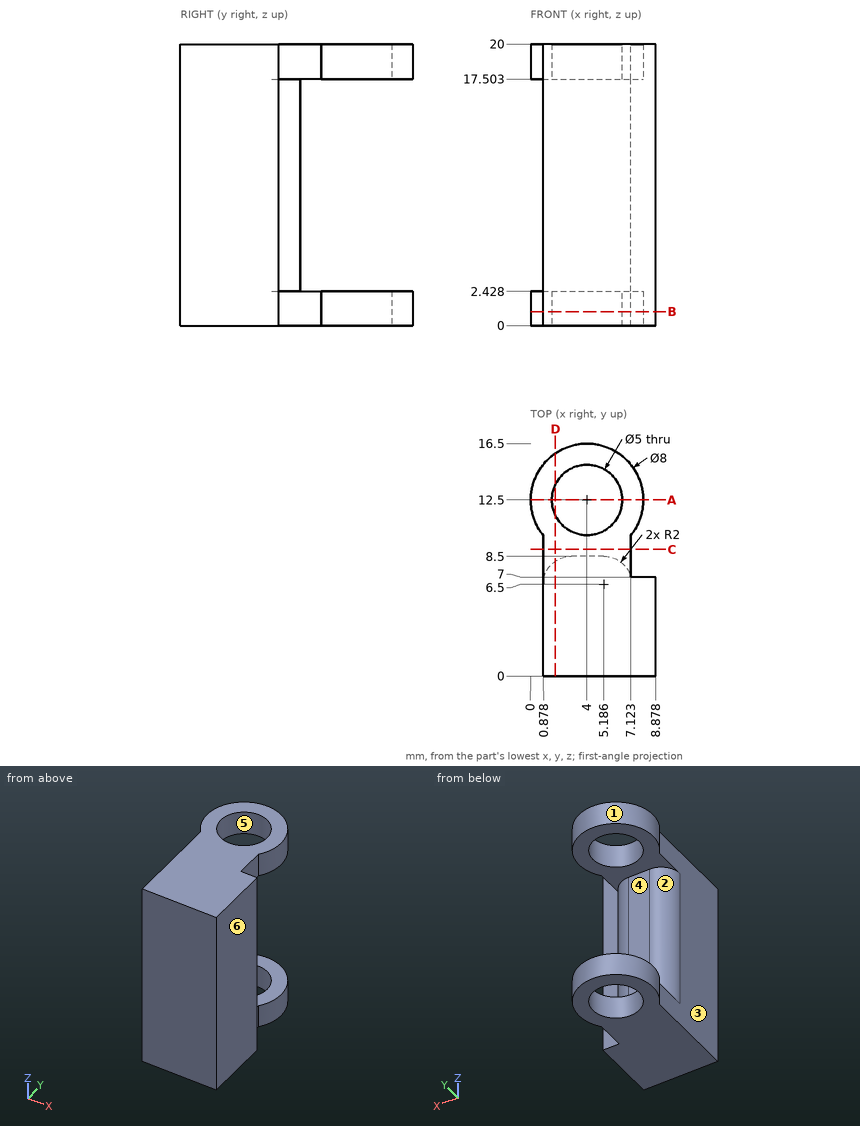
Geometry: see drawing. Coordinates: mm, zero at the bounding-box minimum. A direction names the side the tool comes from. Coordinates: 2 decimals unless noted, no trailing zeros. Loops run counter-clockwise (first coordinate to the right, second up) from the corner with the lowest first, then second, coordinate; pieces in that order, holes last.
(1) First-contact query: pin 1 Ø4 at (x, z) = (5, 7) entering from +Y; pin 2 Ø0.7 at (y, z) = (8, 0.5) entering from +X; pin 3 Ø4 at (x, y) = (4, 11) entering from +Z; pin 4 Ø1.4 at (x, z) = (7.5, 5.5) entering from +Y. Flat tips, straight axial feed; report the tip coordinate or a pass-through.
(2) Set-up query: the marked faces 1, 2 and 3. Return all of +Z, -Z, +X, -X, +Y, -Y with unobstructed straight access to the full face (end or side cutting, diameter ignored); none if empty.
(3) Section A-A on y = 12.5. Return the cut outline in (x, z).
(4) Pull-direction query (X, two-part tool) for the marked faces 4, 5 and 6; classes: released by +X, released by -X, zero draft, split by the parting line, or undercut.
(5) Section D-D on x = 1.75. Return the cut outline in (y, z).
(6) Material intervals for probe 1 along Z at (x, y) = (1, 12.75); probe 2 along X at (y, z) = (1, 19); probe 3 along Y at (x, z) = (4, 9), sorted ascending.
(7) Section B-B on z = 1. Return the cut outline in (x, y).
(8) Section C-C on y = 9. Return the cut outline in (x, z).
Data:
1. pin 1: stops at y = 8.5
1. pin 2: stops at x = 7.12
1. pin 3: stops at z = 20
1. pin 4: stops at y = 7.68
2. face 1: +Z, -Z
2. face 2: -X, +Y
2. face 3: +Z, -Z, -X, -Y
3. outline: (0, 0) - (1.5, 0) - (1.5, 2.43) - (0, 2.43) - close; (0, 17.5) - (1.5, 17.5) - (1.5, 20) - (0, 20) - close; (6.5, 0) - (8, 0) - (8, 2.43) - (6.5, 2.43) - close; (6.5, 17.5) - (8, 17.5) - (8, 20) - (6.5, 20) - close
4. face 4: zero draft
4. face 5: undercut
4. face 6: released by +X
5. outline: (0, 0) - (11.41, 0) - (11.41, 2.43) - (8.15, 2.43) - (8.15, 17.5) - (11.41, 17.5) - (11.41, 20) - (0, 20) - close; (13.59, 0) - (15.81, 0) - (15.81, 2.43) - (13.59, 2.43) - close; (13.59, 17.5) - (15.81, 17.5) - (15.81, 20) - (13.59, 20) - close
6. probe 1: z = 0 to 2.43, 17.5 to 20
6. probe 2: x = 0.88 to 8.88
6. probe 3: y = 0 to 8.5
7. outline: (0.88, 0) - (8.88, 0) - (8.88, 7) - (7.12, 7) - (7.12, 10) arc R4 ccw (long way) to (0.88, 10) - close; hole circle Ø5 at (4, 12.5)
8. outline: (0.88, 0) - (7.12, 0) - (7.12, 2.43) - (0.88, 2.43) - close; (0.88, 17.5) - (7.12, 17.5) - (7.12, 20) - (0.88, 20) - close
